For this review, take the finished solid that the model builds, in its own axes (mm). Face numbers are marked on the shaded views. A direction names the side the tool comes from. Coordinates: 2 decimals unless noted, no trailing zeros. Write each loop counter-clockwise with the first axis right and the second up, starting at its lowest first coordinate (ties: lowest second). Pieces come first, ordered by that corner, then holes. Notation, with made-up numbers: M 87,-10 L 109,-10 A22 ccw 109,16 Z; hole C -21,60.25 d7. An arc over 180 degrees is marked long. One line per question, with ' | ' between items.
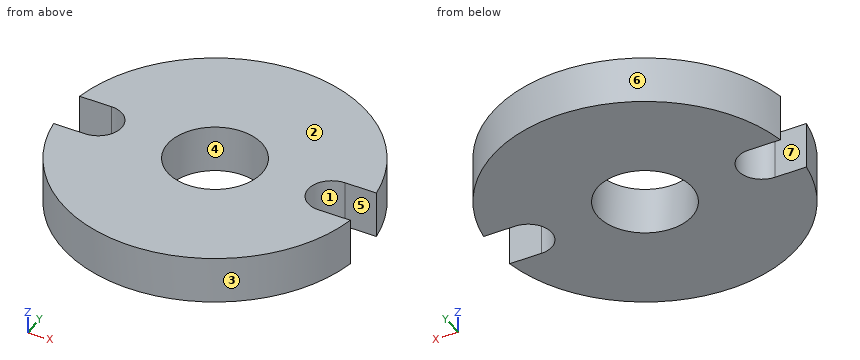
from build123d import *

# Parameters (mm, degrees)
SKETCH_1_R      = 1.5
EXTRUDE_1_DEPTH = 1.5


with BuildPart() as part:
    # Эскиз1 → Бобышка-Вытянуть1 (new body)
    with BuildSketch(Plane.XY):
        with BuildLine():
            ThreePointArc((4.766353428, 0.75), (0, 4.825), (-4.766353428, 0.75))
            Line((-4.766353428, 0.75), (-3.75, 0.75))
            ThreePointArc((-3.75, 0.75), (-3, 0), (-3.75, -0.75))
            Line((-3.75, -0.75), (-4.766353428, -0.75))
            ThreePointArc((-4.766353428, -0.75), (0, -4.825), (4.766353428, -0.75))
            Line((4.766353428, -0.75), (3.75, -0.75))
            ThreePointArc((3.75, -0.75), (3, 0), (3.75, 0.75))
            Line((3.75, 0.75), (4.766353428, 0.75))
        make_face()
        Circle(SKETCH_1_R, mode=Mode.SUBTRACT)
    extrude(amount=EXTRUDE_1_DEPTH)


solid = part.part
1. Machinability: for the marked faces 5, 6 and 7, which of the approach directions +Z, -Z, +X, -X, +Y, -Y give a long, thin tool a straight path to every point of the face, cutting with its end or side? Answer none if there is none.
Computed values:
face 5: +Z, -Z, +X | face 6: +Z, -Z, +Y | face 7: +Z, -Z, -X
2. Clearance check with flat-ended pins moving along their axes: P1, Ø0.5, axis at x = -4, z = 0.5, coming from the +Y side; P2, Ø3.5, axis at x = 0, y = 0, coming from the -Z side; P3, Ø0.8, axis at x = 4.5, z = 0.5, coming from the -Y side; P4, Ø0.5, axis at x = -4, z = 1, coming from the -Y side. State where each tip first meets the part, or that it passes through.
Computed values:
P1: stops at y = 3.04 | P2: stops at z = 0 | P3: stops at y = -2.54 | P4: stops at y = -3.04
3. Take a section at D-D on y = -3.25. State the section outline as (x, z) points, plus the area to 3 significant figures.
Computed values:
outline: M -3.57,0 L 3.57,0 L 3.57,1.5 L -3.57,1.5 Z | area: 10.7 mm2
4. Draft analysis for pull direction Y (two halves, no side actions). For the marked faces 1, 2, 3 and 4, state which applies: pulls with the +Y half, pulls with the -Y half, needs draft (parallel to the pull), parting line crosses it, or undercut.
Computed values:
face 1: undercut | face 2: needs draft | face 3: pulls with the -Y half | face 4: undercut
5. For line 1 along Y through (x, z) = (0, 0.55) (3 decimals); line 2 along X through (y, z) = (0.5, 0.5); line 3 along X through (y, z) = (1.25, 0.5), list the stretches that pass through material, from the lowest coordinate up.
Computed values:
line 1: y = -4.825 to -1.5, 1.5 to 4.825 | line 2: x = -3.19 to -1.41, 1.41 to 3.19 | line 3: x = -4.66 to -0.83, 0.83 to 4.66
6. Take a section at B-B on y = 0. State the section outline as (x, z) points, plus the area to 3 significant figures.
Computed values:
outline: M -3,0 L -1.5,0 L -1.5,1.5 L -3,1.5 Z; M 1.5,0 L 3,0 L 3,1.5 L 1.5,1.5 Z | area: 4.50 mm2
7. Take a section at C-C on x = 0. State the section outline as (y, z) points (3 decimals).
Computed values:
outline: M -4.825,0 L -1.5,0 L -1.5,1.5 L -4.825,1.5 Z; M 1.5,0 L 4.825,0 L 4.825,1.5 L 1.5,1.5 Z
8. Take a section at A-A on z = 1.25. State the section outline as (x, y) points (3 decimals), plus the area to 3 significant figures.
Computed values:
outline: M -4.766,-0.75 A4.825 ccw 4.766,-0.75 L 3.75,-0.75 A0.75 cw 3.75,0.75 L 4.766,0.75 A4.825 ccw -4.766,0.75 L -3.75,0.75 A0.75 cw -3.75,-0.75 Z; hole C 0,0 d3 | area: 61.1 mm2
